Source: CAD feature listing. Evaluate the final solid. Frame: model axes, mm. A direction names the side the tool comes from. Coordinates: 2 decimals unless noted, no trailing zeros. Order: outer loops, then holes, each group sorted by start corner. A loop starts at its lowest first (then second) coordinate and runs counter-clockwise, first axis right, second up.
```python
from build123d import *

# Parameters (mm, degrees)
F0_R     = 1.905
F1_DEPTH = 7.62
F2_R     = 21.59
F3_DEPTH = 25.4
F4_R     = 5.08


with BuildPart() as f1:
    # F0 (on Front) → F1 (new body)
    with BuildSketch(Plane.XZ):
        Circle(F0_R)
    extrude(amount=F1_DEPTH)

    # F2 (on face) → F3 (join)
    with BuildSketch(Plane.XZ.offset(7.62)):
        Circle(F2_R)
    extrude(amount=F3_DEPTH)

    # F4
    f4_edges = [f1.edges().sort_by_distance(p)[0] for p in [
        (-21.59, -33.02, 0),
        (-21.59, -7.62, 0),
    ]]
    fillet(f4_edges, radius=F4_R)


solid = f1.part
```
1. Section query C-C, the plane y = -7. Output: boundary loops of the cut face in (x, z) (3 decimals), plus the area to 3 significant figures.
2. Section query D-D, the plane y = -16.5. Output: boundary loops of the cut face in (x, z), plus the area to 3 significant figures.
3. Access query for faces 1 (the cylindrical face through (-0.41, -3.76, -1.86)), 2 (the flat face through (0, -33.02, 0)). Directions: +Z, -Z, +X, -X, +Y, -Y. A direction counts if a zero-diameter tool reaches every point of the face in a straight line with its end or side. Return the directions, or none.
4. Material intervals for line 1 along Y through (x, z) = (8, -4); line 2 along X through (y, z) = (-11, -7); line 3 along Z through (x, y) = (0, -29.5), sorted ascending.
5. Section query A-A, the plane x = 0. Output: boundary loops of the cut face in (y, z) (3 decimals).
6. Section query B-B, the plane z = 0. Output: boundary loops of the cut face in (x, y) (3 decimals), plus the area to 3 significant figures.
7. Contact query for flat-ended pins moving along their axis: P1, Ø8, axis at y = -26.5, z = 13, coming from the -X side; P2, Ø3, axis at x = -3.5, y = -10.5, coming from the +Z side; P3, Ø12, axis at x = 4.5, z = 12, coming from the +Y side. Output: stop coordinate, or through.
Answer key:
1. outline: circle Ø3.81 at (0, 0)
1. area: 11.4 mm2
2. outline: circle Ø43.18 at (0, 0)
2. area: 1,460 mm2
3. face 1: +Y
3. face 2: +Z, -Z, +X, -X, -Y
4. line 1: y = -33.02 to -7.62
4. line 2: x = -20.11 to 20.11
4. line 3: z = -21.34 to 21.34
5. outline: (-33.02, -16.51) arc R5.08 ccw to (-27.94, -21.59) - (-12.7, -21.59) arc R5.08 ccw to (-7.62, -16.51) - (-7.62, -1.905) - (0, -1.905) - (0, 1.905) - (-7.62, 1.905) - (-7.62, 16.51) arc R5.08 ccw to (-12.7, 21.59) - (-27.94, 21.59) arc R5.08 ccw to (-33.02, 16.51) - close
6. outline: (-21.59, -27.94) arc R5.08 ccw to (-16.51, -33.02) - (16.51, -33.02) arc R5.08 ccw to (21.59, -27.94) - (21.59, -12.7) arc R5.08 ccw to (16.51, -7.62) - (1.905, -7.62) - (1.905, 0) - (-1.905, 0) - (-1.905, -7.62) - (-16.51, -7.62) arc R5.08 ccw to (-21.59, -12.7) - close
6. area: 1,100 mm2
7. P1: stops at x = -19.62
7. P2: stops at z = 21.33
7. P3: stops at y = -7.62
